CAD build for the part. Positions are in the model's coordinates, mm. Face numbers are marked on the shaded views. A direction names the side the tool comes from. Round coordinates to 2 decimals unless told otherwise and drop trailing zeros. Loops run counter-clockwise (first coordinate to the right, second up) from the corner with the lowest first, then second, coordinate; pieces in that order, holes last. Notation, with made-up numbers: (-21, -24.5) -> (0, -24.5) arc R21 ccw to (0, -16.5) -> close; hole circle Ø7 at (8, 28). An arc over 180 degrees is marked (long way). Answer as CSV lines item,"result".
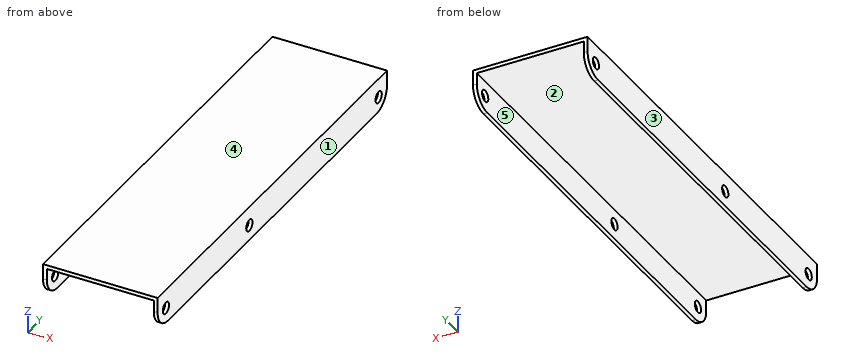
```python
from build123d import *

# Parameters (mm, degrees)
F1_DEPTH = 110
F2_R     = 1.5
F3_DEPTH = 35
F4_R     = 5


with BuildPart() as f1:
    # F0 (on Front) → F1 (new body)
    with BuildSketch(Plane.XZ):
        Polygon((15, 0), (-15, 0), (-15, -9), (-14, -9), (-14, -1), (14, -1), (14, -9), (15, -9), align=None)
    extrude(amount=F1_DEPTH)

    # F2 (on face) → F3 (cut)
    with BuildSketch(Plane.YZ.offset(15)):
        with Locations((-106, -5)):
            Circle(F2_R)
        with Locations((-66, -5)):
            Circle(F2_R)
        with Locations((-4, -5)):
            Circle(F2_R)
    extrude(amount=-F3_DEPTH, mode=Mode.SUBTRACT)

    # F4
    f4_edges = [f1.edges().sort_by_distance(p)[0] for p in [
        (14.5, -110, -9),
        (-14.5, -110, -9),
        (14.5, 0, -9),
        (-14.5, 0, -9),
    ]]
    fillet(f4_edges, radius=F4_R)


solid = f1.part
```
Q1. Slice it at D-D, the plane x = -6. Give the cut face in (y, z).
Results:
outline,"(-110, -1) -> (0, -1) -> (0, 0) -> (-110, 0) -> close"
Q2. Probe L1, parallel to X at y = -46.5, z = -7.25; L2, parallel to Z at x = -3.5, y = -34; L3, parallel to Z at x = -14.45, y = -66. List the from-to ranges inside material, lowest first. Write a range as [from, to].
Results:
L1,"[-15, -14], [14, 15]"
L2,"[-1, 0]"
L3,"[-9, -6.5], [-3.5, 0]"
Q3. Two-plate mould, pull along X, no slides. Class the marked faces 3, 4 and 5: pulls with the +X half, pulls with the -X half, needs draft (parallel to the pull), parting line crosses it, or undercut.
Results:
face 3,"pulls with the -X half"
face 4,"needs draft"
face 5,"undercut"
Q4. Slice it at A-A, the plane y = -66. Give the cut face in (x, z).
Results:
outline,"(-15, -9) -> (-14, -9) -> (-14, -6.5) -> (-15, -6.5) -> close; (-15, -3.5) -> (-14, -3.5) -> (-14, -1) -> (14, -1) -> (14, -3.5) -> (15, -3.5) -> (15, 0) -> (-15, 0) -> close; (14, -9) -> (15, -9) -> (15, -6.5) -> (14, -6.5) -> close"
Q5. Slice it at B-B, the plane z = -5. Count the separate pieces of the cut face and the enclosed holes in it, and give its area (3 significant figures).
Results:
separate pieces,"8"
enclosed holes,"0"
area,"202 mm2"
Q6. Slice it at C-C, the plane y = -106. Give the cut face in (x, z), and give its area (3 significant figures).
Results:
outline,"(-15, -8.9) -> (-14, -8.9) -> (-14, -6.5) -> (-15, -6.5) -> close; (-15, -3.5) -> (-14, -3.5) -> (-14, -1) -> (14, -1) -> (14, -3.5) -> (15, -3.5) -> (15, 0) -> (-15, 0) -> close; (14, -8.9) -> (15, -8.9) -> (15, -6.5) -> (14, -6.5) -> close"
area,"39.8 mm2"
Q7. Tool access for the marked faces 1 and 2: list every direction of +Z, -Z, +X, -X, +Y, -Y with a clear straight run to the whole face (end or side of a thin tool).
Results:
face 1,"+Z, -Z, +X, +Y, -Y"
face 2,"-Z, +Y, -Y"
Q8. Drop flat-ended pins along their axis: pin 1 Ø8 at (x, y) = (11.5, -92) entering from +Z; pin 2 Ø5 at (x, y) = (5, -86) entering from -Z. Give the stop position or say it passes through.
Results:
pin 1,"z = 0"
pin 2,"z = -1"
